```python
from build123d import *

# Parameters (mm, degrees)
F2_R   = 20
F2_R_2 = 18


with BuildPart() as f3:
    # F3: sweep along a path in F0
    with BuildLine(Plane.XZ) as f3_path:
        Line((0, 350), (0, 200))
        ThreePointArc((0, 200), (58.578644, 58.578644), (200, 0))
        Line((200, 0), (350, 0))
    # F2 (on plane+point) → F3 (sweep)
    with BuildSketch(Plane.XY.offset(350)):
        Circle(F2_R)
        Circle(F2_R_2, mode=Mode.SUBTRACT)
    sweep(path=f3_path.line)


solid = f3.part
```
The model under review builds one solid part; all positions refer to its coordinate system, in mm. Give positions to 0.01 mm unless a question says otherwise; leave off trailing zeros. Write each loop counter-clockwise with the first axis right and the second up, starting at its lowest first coordinate (ties: lowest second). Pieces come first, ordered by that corner, then holes. Notation, with made-up numbers: (14.25, -28) -> (53.25, -28) arc R6 ccw to (53.25, -19) -> close; hole circle Ø1 at (46, 14). An arc over 180 degrees is marked (long way). Put each result on its own line as item: value.
(1) The part is to be moulded in two halves that separate along X. For faces 1 (the cylindrical face through (-2.343, -17.847, 273.95)), 2 (the cylindrical face through (-4.336, 19.524, 273.95)), 3 (the flat face through (-18, 3, 350)), say which applies: pulls with the +X half, pulls with the -X half, needs draft (parallel to the pull), parting line crosses it, or undercut.
Results are:
face 1: undercut
face 2: parting line crosses it
face 3: needs draft
(2) For pin 1 Ø2 at (y, z) = (-12.5, 212.5) entering from -X; pin 2 Ø10 at (y, z) = (16, 185.5) entering from -X; pin 3 Ø2 at (x, y) = (91, -6) entering from +Z, all flat-tipped, find the tip position at first contact; note any pin that passes through.
Results are:
pin 1: x = -16.36
pin 2: x = -16.23
pin 3: z = 56.45
(3) To check wall thickness, follow probe 1 along Y at (x, z) = (0, 272); probe 2 along Z at (x, y) = (46.5, -5). State the ranges of each line that lie inside material, in increasing order. Write a range as from..to.
Results are:
probe 1: -20..-18, 18..20
probe 2: 43.29..46.2, 100.9..104.78
(4) We need section A-A, the plane z = 243. Give the boundary of the cut face in (x, y), and give its area (3 significant figures).
Results are:
outline: circle Ø40 at (0, 0); hole circle Ø36 at (0, 0)
area: 239 mm²
